```python
from build123d import *

# Parameters (mm, degrees)
SKETCH1_R           = 80
SKETCH1_R_2         = 6
BOSS_EXTRUDE1_DEPTH = 13
SKETCH2_R           = 65
CUT_EXTRUDE1_DEPTH  = 8
SKETCH5_R           = 13
SKETCH5_R_2         = 6
BOSS_EXTRUDE2_DEPTH = 18
CHAMFER1_SIZE       = 1
CUT_EXTRUDE2_DEPTH  = 116.451288429
CIRPATTERN1_COUNT   = 8


with BuildPart() as part:
    # Sketch1 → Boss-Extrude1 (new, symmetric)
    with BuildSketch(Plane.XY):
        with Locations(Location((0, 0, 0), (0, 0, 180))):
            Circle(SKETCH1_R)
        with Locations(Location((0, 0, 0), (0, 0, 180))):
            Circle(SKETCH1_R_2, mode=Mode.SUBTRACT)
    extrude(amount=BOSS_EXTRUDE1_DEPTH, both=True)

    # Sketch2 → Cut-Extrude1 (cut)
    with BuildSketch(Plane.XY.offset(13)):
        Circle(SKETCH2_R)
    cut_extrude1 = extrude(amount=-CUT_EXTRUDE1_DEPTH, mode=Mode.SUBTRACT)

    # Mirror1: Cut-Extrude1 across plane
    add(cut_extrude1.mirror(Plane.XY), mode=Mode.SUBTRACT)

    # Sketch5 → Boss-Extrude2 (add, symmetric)
    with BuildSketch(Plane.XY):
        with Locations(Location((0, 0, 0), (0, 0, 180))):
            Circle(SKETCH5_R)
        with Locations(Location((0, 0, 0), (0, 0, 180))):
            Circle(SKETCH5_R_2, mode=Mode.SUBTRACT)
    extrude(amount=BOSS_EXTRUDE2_DEPTH, both=True)

    # Chamfer1
    chamfer1_edges = [part.edges().sort_by_distance(p)[0] for p in [
        (-65, 0, 13),
        (-65, 0, -13),
        (80, 0, -13),
        (80, 0, 13),
    ]]
    chamfer(chamfer1_edges, length=CHAMFER1_SIZE)

    # Sketch7 → Cut-Extrude2 (cut, symmetric)
    with BuildSketch(Plane.XY.offset(5)):
        with BuildLine():
            Line((0, 54.772255751), (0, 19.397164741))
            ThreePointArc((0, 19.397164741), (-0.515032591, 18.057436487), (-1.794871795, 17.407711947))
            ThreePointArc((-1.794871795, 17.407711947), (-4.529333289, 16.90370196), (-7.149451403, 15.972956666))
            ThreePointArc((-7.149451403, 15.972956666), (-8.582686936, 15.895715021), (-9.698582371, 16.798437427))
            Line((-9.698582371, 16.798437427), (-27.386127875, 47.434164903))
            ThreePointArc((-27.386127875, 47.434164903), (-27.821744262, 51.446675992), (-25.152000934, 54.473634439))
            ThreePointArc((-25.152000934, 54.473634439), (-15.529142706, 57.955549577), (-5.454545455, 59.751551728))
            ThreePointArc((-5.454545455, 59.751551728), (-1.629000688, 58.46500048), (0, 54.772255751))
        make_face()
    cut_extrude2 = extrude(amount=CUT_EXTRUDE2_DEPTH, both=True, mode=Mode.SUBTRACT)

    # CirPattern1: Cut-Extrude2 ×8 about axis
    cirpattern1_axis = Axis((0, 0, 0), (0, 0, 1))
    for i in range(1, CIRPATTERN1_COUNT):
        add(cut_extrude2.rotate(cirpattern1_axis, i * 360 / CIRPATTERN1_COUNT), mode=Mode.SUBTRACT)


solid = part.part
```
Verification items for the finished model (mm, model axes). A direction names the side the tool comes from. Give positions to 0.01 mm unless a question says otherwise; leave off trailing zeros. Loops run counter-clockwise (first coordinate to the right, second up) from the corner with the lowest first, then second, coordinate; pieces in that order, holes last. Notation, with made-up numbers: M 80,-17 L 112,-17 A7 ccw 112,-8 Z; hole C -6.75,9.5 d8. An arc over 180 degrees is marked long. One line per question, with ' | ' between items.
Item 1: Depth check by flat-ended pin: P1, Ø3, axis at x = -45, z = 1.5, coming from the -Y side; P2, Ø11, axis at y = 30, z = 1.5, coming from the -X side; P3, Ø6, axis at x = 43, z = -9, coming from the -Y side; P4, Ø5, axis at x = -18.5, y = 39, coming from the -Z side. Enter the tip coordinate at first touch or a pass-through.
Completed:
P1: stops at y = -67.14 | P2: stops at x = -76.16 | P3: stops at y = -69.28 | P4: passes through
Item 2: Section check C-C, the plane y = 36. State how many separate pieces and enclosed holes the cut face has, plus the area to 3 significant figures.
Completed:
separate pieces: 4 | enclosed holes: 0 | area: 1,390 mm^2
Item 3: Thickness scan on line 1 (Y direction, x = 0, z = -8.75); line 2 (Y direction, x = 30, z = -1); line 3 (X direction, y = -3, z = 10.5). Record the ranges inside material, lowest first. Write a range as [from, to].
Completed:
line 1: y = [-80, -65], [-13, -6], [6, 13], [65, 80] | line 2: y = [-74.16, -30], [-8.04, 0], [17.32, 30], [51.96, 74.16] | line 3: x = [-79.94, -64.93], [-12.65, -5.2], [5.2, 12.65], [64.93, 79.94]
Item 4: Section check B-B, the plane z = 9.5. Record the cut outline in (x, y), plus the area to 3 significant figures.
Completed:
outline: C 0,0 d160; C 0,0 d26; hole C 0,0 d130; hole C 0,0 d12 | area: 7,250 mm^2
Item 5: Tool access check on faces 1 (the face through (-1, -14, -5)), 2 (the face through (-58.5, -1.67, 0.07)). Record the directions out of +Z, -Z, +X, -X, +Y, -Y that give a thin tool (end or side, any length) a straight path to the whole face; none if there is none.
Completed:
face 1: -Z | face 2: +Z, -Z
Item 6: Section check A-A, the plane z = -15.5. Record the cut outline in (x, y).
Completed:
outline: C 0,0 d26; hole C 0,0 d12
